```python
from build123d import *

# Parameters (mm, degrees)
SKETCH1_W               = 3.5
SKETCH1_H               = 3.5
BOSS_EXTRUDE1_DEPTH     = 14
CUT_EXTRUDE1_DEPTH      = 1.5
CUT_EXTRUDE1_DEPTH_BACK = 1.5


with BuildPart() as part:
    # Sketch1 → Boss-Extrude1 (new body)
    with BuildSketch(Plane.XY):
        Rectangle(SKETCH1_W, SKETCH1_H)
    extrude(amount=BOSS_EXTRUDE1_DEPTH)

    # Sketch2 → Cut-Extrude1 (cut, two sides)
    with BuildSketch(Plane.XY.offset(7)) as cut_extrude1_sk:
        with BuildLine():
            Line((1.75, -1.75), (1.75, 0))
            ThreePointArc((1.75, 0), (0.512563133, 0.512563133), (0, 1.75))
            Line((0, 1.75), (-1.75, 1.75))
            Line((-1.75, 1.75), (-1.75, -1.75))
            Line((-1.75, -1.75), (1.75, -1.75))
        make_face()
    extrude(amount=CUT_EXTRUDE1_DEPTH, mode=Mode.SUBTRACT)
    extrude(cut_extrude1_sk.sketch, amount=-CUT_EXTRUDE1_DEPTH_BACK, mode=Mode.SUBTRACT)


solid = part.part
```
The listing builds one solid part. Answer for the finished solid, in the listing's coordinates (mm). A direction names the side the tool comes from. Give positions to 0.01 mm unless a question says otherwise; leave off trailing zeros. Write each loop counter-clockwise with the first axis right and the second up, starting at its lowest first coordinate (ties: lowest second). Pieces come first, ordered by that corner, then holes. Notation, with made-up numbers: (-31, 53) - (1, 53) arc R33 ccw to (1, 88) - close; hole circle Ø10 at (41.25, 59). An arc over 180 degrees is marked (long way). Use one line per item in the form item = value. Start each with the question number.
1) Find section D-D on z = 7.25. Determine the outline of the cut face in (x, y).
2) The mould has two halves that part along Z. Classify faces 3 (the face through (-1.75, 0, 3)), 4 (the face through (0, 0, 8.5)), 5 (the face through (0, 0, 0)), 6 (the face through (0, 0, 14)): pulls with the +Z half, pulls with the -Z half, needs draft (parallel to the pull), parting line crosses it, or undercut.
3) Consider line 1 along Z through (x, y) = (-0.9, -0.45); line 2 along Y through (x, z) = (0.5, 6.25); line 3 along Y through (x, z) = (0.7, 7.5). Determine where each line is inside the solid, lowest interval first. Write a range as from..to.
4) Find section A-A on x = -1.35. Determine the outline of the cut face in (y, z).
5) Find section C-C on x = 0.65. Determine the outline of the cut face in (y, z), plus the area to 3 significant figures.
6) A tool of negligible diameter and unlimited length cuts with its end or side. For faces 1 (the face through (0, -1.75, 3)), 2 (the face through (0.526, 0.499, 6.979)), from which of +Z, -Z, +X, -X, +Y, -Y can it reach the whole face along a straight path? Write none if from no direction.
Geometry results:
q1.outline = (0, 1.75) arc R1.75 ccw to (1.75, 0) - (1.75, 1.75) - close
q2.face_3 = needs draft
q2.face_4 = undercut
q2.face_5 = pulls with the -Z half
q2.face_6 = pulls with the +Z half
q3.line_1 = 0..5.5, 8.5..14
q3.line_2 = 0.53..1.75
q3.line_3 = 0.35..1.75
q4.outline = (-1.75, 0) - (1.75, 0) - (1.75, 5.5) - (-1.75, 5.5) - close; (-1.75, 8.5) - (1.75, 8.5) - (1.75, 14) - (-1.75, 14) - close
q5.outline = (-1.75, 0) - (1.75, 0) - (1.75, 14) - (-1.75, 14) - (-1.75, 8.5) - (0.39, 8.5) - (0.39, 5.5) - (-1.75, 5.5) - close
q5.area = 42.6 mm2
q6.face_1 = +Z, -Z, +X, -X, -Y
q6.face_2 = -X, -Y
